from build123d import *

# Parameters (mm, degrees)
BOSS_EXTRUDE1_DEPTH = 2.25
FILLET1_R           = 5
SKETCH2_R           = 1.75
CUT_EXTRUDE1_DEPTH  = 48.810012982
BOSS_EXTRUDE2_REACH = 42.044
SKETCH4_W           = 7.5
SKETCH4_H           = 2.1
SKETCH4_2_W         = 7.5
SKETCH4_2_H         = 2.1
BOSS_EXTRUDE3_DEPTH = 1.570511633
FILLET2_R           = 3
FILLET3_R           = 1.2
FILLET4_R           = 0.5


with BuildPart() as part:
    # Sketch1 → Boss-Extrude1 (new body)
    with BuildSketch(Plane(origin=(0, 0, 0), x_dir=(1, 0, 0), z_dir=(0, 1, 0))):
        Polygon((0, 0), (9.481214188, 15.300541739), (17.234295106, 42.205740796), (22.347489461, 42.205740796), (17.140904697, 12.99204844), (7.659690509, -2.308493299), align=None)
    extrude(amount=BOSS_EXTRUDE1_DEPTH)

    # Fillet1
    # the kernel refuses this fillet: 5 mm, written as the material it takes off along each edge
    with BuildSketch(Plane(origin=(7.659690509, -9.589301146, 2.308493299), x_dir=(0.5267341215597666, 0, -0.8500300966346198), z_dir=(0, 1, 0))) as fillet1_piece_1:
        with BuildLine():
            CenterArc((FILLET1_R * 0.767144091705, FILLET1_R), FILLET1_R, 195.013192562, 74.986807438)
            Line((-FILLET1_R * 0.19872211495, FILLET1_R * 0.740958553812), (0, 0))
            Line((0, 0), (FILLET1_R * 0.767144091705, 0))
        make_face()
    extrude(amount=21.428602293, mode=Mode.SUBTRACT)
    with BuildSketch(Plane(origin=(0, -16.294200966, 0), x_dir=(0.5267341215597675, 0, -0.8500300966346193), z_dir=(0, 1, 0))) as fillet1_piece_2:
        with BuildLine():
            CenterArc((FILLET1_R * 1.30353607727, -FILLET1_R), FILLET1_R, 90, 105.013192562)
            Line((FILLET1_R * 0.337669870614, -FILLET1_R * 1.25904144619), (0, 0))
            Line((0, 0), (FILLET1_R * 1.30353607727, 0))
        make_face()
    extrude(amount=34.838401932, mode=Mode.SUBTRACT)

    # Sketch2 → Cut-Extrude1 (cut, through all)
    with BuildSketch(Plane(origin=(0, 2.25, 0), x_dir=(1, 0, 0), z_dir=(0, 1, 0))):
        with Locations(Location((8.167211871, 5.629873064, 0), (0, 0, 270))):
            Circle(SKETCH2_R)
        with Locations(Location((14.031451824, 18.342492377, 0), (0, 0, 270))):
            Circle(SKETCH2_R)
    extrude(amount=-CUT_EXTRUDE1_DEPTH, mode=Mode.SUBTRACT)

    # Boss-Extrude2: up to this plane
    boss_extrude2_end = Plane(origin=(17.140904697, 2.25, -12.99204844), z_dir=(-0.9844866893056965, 0, -0.17545927897922378))
    # Sketch4 → Boss-Extrude2 (add, up to the surface)
    with BuildSketch(Plane(origin=(23.5, -1.484709168, -8.201879583), x_dir=(0, 0, -1), z_dir=(1, 0, 0)), mode=Mode.PRIVATE) as boss_extrude2_sk1:
        with Locations((27.908493587, 2.541926215)):
            Rectangle(SKETCH4_W, SKETCH4_H)
    boss_extrude2_tool1 = split(extrude(boss_extrude2_sk1.sketch, amount=-BOSS_EXTRUDE2_REACH, mode=Mode.PRIVATE), bisect_by=boss_extrude2_end, keep=Keep.BOTH, mode=Mode.PRIVATE)
    add(boss_extrude2_tool1.solids().sort_by_distance((23.5, 1.057217, -36.110373))[0])

    # Sketch4<2> → Boss-Extrude3 (add)
    with BuildSketch(Plane(origin=(23.5, -1.484709168, -8.201879583), x_dir=(0, 0, -1), z_dir=(1, 0, 0))):
        with Locations((27.908493587, 2.541926215)):
            Rectangle(SKETCH4_2_W, SKETCH4_2_H)
    extrude(amount=-BOSS_EXTRUDE3_DEPTH)

    # Fillet2
    fillet2_edges = [part.edges().sort_by_distance(p)[0] for p in [
        (17.234295106, 1.125, -42.205740796),
    ]]
    fillet(fillet2_edges, radius=FILLET2_R)

    # Fillet3
    fillet3_edges = [part.edges().sort_by_distance(p)[0] for p in [
        (22.347489461, 1.125, -42.205740796),
    ]]
    fillet(fillet3_edges, radius=FILLET3_R)

    # Fillet4
    fillet4_edges = [part.edges().sort_by_distance(p)[0] for p in [
        (23.5, 1.057217047, -39.86037317),
        (23.5, 1.057217047, -32.36037317),
    ]]
    fillet(fillet4_edges, radius=FILLET4_R)


solid = part.part
The listing builds one solid part. Answer for the finished solid, in the listing's coordinates (mm). A direction names the side the tool comes from. Coordinates: 2 decimals unless noted, no trailing zeros. Write each loop counter-clockwise with the first axis right and the second up, starting at its lowest first coordinate (ties: lowest second). Pieces come first, ordered by that corner, then holes. Notation, with made-up numbers: (-3.75, 32.25) - (22.25, 32.25) arc R26 cw to (22.25, 51.25) - close; hole circle Ø10 at (21.5, -17). An arc over 180 degrees is marked (long way). Return JSON: item names as keys, results as strings.
1. Consider line 1 along X through (y, z) = (1.15, -5.5); line 2 along X through (y, z) = (0.2, -17.5); line 3 along Z through (x, y) = (8.25, 1.4). Determine where each line is inside the solid, lowest interval first.
Final values:
{"line 1": "3.41 to 6.42, 9.91 to 12.5", "line 2": "10.12 to 12.5, 15.57 to 17.94", "line 3": "-13.31 to -7.38, -3.88 to 0.54"}
2. Each of these flat-tipped pins is pushed along its axis until it touches: pin 1 Ø1 at (x, y) = (21.5, 0.5) entering from -Z; pin 2 Ø0.5 at (x, y) = (22.5, 1) entering from -Z; pin 3 Ø1.5 at (x, z) = (22.5, -35) entering from +Y. Where does it stop, or does it pass through?
Final values:
{"pin 1": "z = -42.2", "pin 2": "z = -39.86", "pin 3": "y = 2.11"}
3. The part is cut by section B-B on y = 1.4. Determine the outline of the cut face in (x, z).
Final values:
{"outline": "(3.43, -5.54) - (9.48, -15.3) - (16.61, -40.04) arc R3 ccw to (19.49, -42.21) - (20.91, -42.21) arc R1.2 ccw to (22.1, -40.8) - (21.93, -39.86) - (23, -39.86) arc R0.5 ccw to (23.5, -39.36) - (23.5, -32.86) arc R0.5 ccw to (23, -32.36) - (20.59, -32.36) - (17.14, -12.99) - (9.68, -0.95) arc R5 ccw to (5.15, 1.41) arc R5 ccw to start; hole circle Ø3.5 at (8.17, -5.63); hole circle Ø3.5 at (14.03, -18.34)"}
4. The part is cut by section D-D on z = -31.5. Determine the outline of the cut face in (x, y), then the cut area to 3 significant figures.
Final values:
{"outline": "(14.15, 0) - (20.44, 0) - (20.44, 2.25) - (14.15, 2.25) - close", "area": "14.2 mm^2"}
5. The part is cut by section A-A on z = -18. Determine the outline of the cut face in (x, y).
Final values:
{"outline": "(10.26, 0) - (12.32, 0) - (12.32, 2.25) - (10.26, 2.25) - close; (15.75, 0) - (18.03, 0) - (18.03, 2.25) - (15.75, 2.25) - close"}
6. Which of the six approach directions +Z, -Z, +X, -X, +Y, -Y give full straight-line access (tool end or side, diameter ignored) to faces 1 (the face through (22, 1, -32.36)), 2 (the face through (13, 2.25, -21))?
Final values:
{"face 1": "+Z, +X, +Y, -Y", "face 2": "+Z, -Z, +X, -X, +Y"}
7. For a pull along Z with two mould halves and no side action, classify faces 3 (the face through (17.67, 1.14, -41.59)), 4 (the face through (15.507, 1.141, -17.402)), 5 (the face through (13.463, 1.109, -7.056)), 6 (the face through (22, 2.107, -36)) as +Z half, -Z half, draft (parallel to the pull), parting line (faces both ways), or undercut.
Final values:
{"face 3": "-Z half", "face 4": "undercut", "face 5": "+Z half", "face 6": "draft"}
